from build123d import *

# Parameters (mm, degrees)
ESTRUSIONE_ESTRUSIONE1_DEPTH = 50
ESTRUSIONE_ESTRUSIONE4_DEPTH = 50
SCHIZZO5_W                   = 50
SCHIZZO5_H                   = 50
ESTRUSIONE_ESTRUSIONE5_DEPTH = 680
SCHIZZO6_W                   = 50
SCHIZZO6_H                   = 50
ESTRUSIONE_ESTRUSIONE6_DEPTH = 150


with BuildPart() as part:
    # Schizzo1 → Estrusione-Estrusione1 (new body)
    with BuildSketch(Plane.XY):
        Polygon((0, 0), (1150, 0), (1150, -1150), (810, -1150), (570, -960), (0, -960), align=None)
        Polygon((50, -50), (1100, -50), (1100, -1100), (827.395936132, -1100), (587.395936132, -910), (50, -910), align=None, mode=Mode.SUBTRACT)
    extrude(amount=ESTRUSIONE_ESTRUSIONE1_DEPTH)



with BuildPart() as body_2:
    # Schizzo4 → Estrusione-Estrusione4 (new body)
    with BuildSketch(Plane(origin=(0, 0, 780), x_dir=(-1, 0, 0), z_dir=(0, 0, -1))):
        Polygon((-1150, -1150), (-810, -1150), (-570, -960), (0, -960), (0, 0), (-1150, 0), align=None)
        Polygon((-50, -50), (-1100, -50), (-1100, -1100), (-827.395936132, -1100), (-587.395936132, -910), (-50, -910), align=None, mode=Mode.SUBTRACT)
    extrude(amount=ESTRUSIONE_ESTRUSIONE4_DEPTH)


with BuildPart() as part_1:
    add(part.part)

    add(body_2.part)  # Estrusione-Estrusione5 merges body 2
    # Schizzo5 → Estrusione-Estrusione5 (add)
    with BuildSketch(Plane(origin=(0, 0, 730), x_dir=(-1, 0, 0), z_dir=(0, 0, -1))):
        with Locations((-1125, -25)):
            Rectangle(SCHIZZO5_W, SCHIZZO5_H)
        with Locations((-25, -25)):
            Rectangle(SCHIZZO5_W, SCHIZZO5_H)
        with Locations((-25, -935)):
            Rectangle(SCHIZZO5_W, SCHIZZO5_H)
        with Locations((-1125, -1125)):
            Rectangle(SCHIZZO5_W, SCHIZZO5_H)
    extrude(amount=ESTRUSIONE_ESTRUSIONE5_DEPTH)

    # Schizzo6 → Estrusione-Estrusione6 (add)
    with BuildSketch(Plane(origin=(0, 0, 0), x_dir=(-1, 0, 0), z_dir=(0, 0, -1))):
        with Locations((-25, -935)):
            Rectangle(SCHIZZO6_W, SCHIZZO6_H)
        with Locations((-1125, -1125)):
            Rectangle(SCHIZZO6_W, SCHIZZO6_H)
        with Locations((-1125, -25)):
            Rectangle(SCHIZZO6_W, SCHIZZO6_H)
        with Locations((-25, -25)):
            Rectangle(SCHIZZO6_W, SCHIZZO6_H)
    extrude(amount=ESTRUSIONE_ESTRUSIONE6_DEPTH)


solid = part_1.part
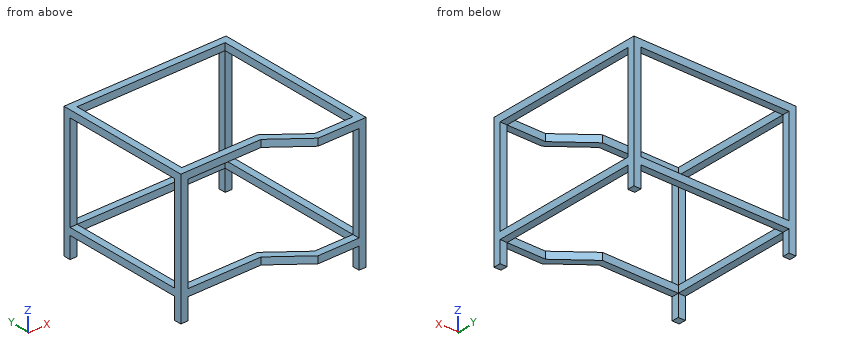
The model under review builds one solid part; all positions refer to its coordinate system, in mm. Give positions to 0.01 mm unless a question says otherwise; leave off trailing zeros. Write each loop counter-clockwise with the first axis right and the second up, starting at its lowest first coordinate (ties: lowest second). Pieces come first, ordered by that corner, then holes. Notation, with made-up numbers: M 75,26 L 87,26 A12 ccw 87,44 Z; hole C 9,-10.75 d6. An arc over 180 degrees is marked long. One line per question, with ' | ' between items. Start each with the question number.
Item 1: Wall thickness on line 1 (X direction, y = -857, z = 29); line 2 (Y direction, x = 669, z = 35) (3 decimals): over which ranges is each line inside the solid? List them lowest first. Write a range as from..to.
Item 2: We need section B-B on z = 100. Write out the cut boundary in (x, y).
Item 3: For pin 1 (25 mm diameter, centred on x = 1129, y = -648, fed in from -Z), flat-tipped, find the tip position at first contact; note if it passes through.
Item 4: We need section A-A on y = -285.5. Write out the cut boundary in (x, z), plus the area to 3 significant figures.
Results found:
1) line 1: x = 0..50, 1100..1150 | line 2: y = -1038.375..-974.603, -50..0
2) outline: M 0,-960 L 50,-960 L 50,-910 L 0,-910 Z; M 0,-50 L 50,-50 L 50,0 L 0,0 Z; M 1100,-1150 L 1150,-1150 L 1150,-1100 L 1100,-1100 Z; M 1100,-50 L 1150,-50 L 1150,0 L 1100,0 Z
3) pin 1: stops at z = 0
4) outline: M 0,0 L 50,0 L 50,50 L 0,50 Z; M 0,730 L 50,730 L 50,780 L 0,780 Z; M 1100,0 L 1150,0 L 1150,50 L 1100,50 Z; M 1100,730 L 1150,730 L 1150,780 L 1100,780 Z | area: 10,000 mm2
